Autodesk Inventor part; units mm, degrees
ref_plane "YZ Plane" through (0, 0, 0) normal (1, 0, 0) x (0, 1, 0)
ref_plane "XZ Plane" through (0, 0, 0) normal (0, 1, 0) x (-1, 0, 0)
ref_plane "XY Plane" through (0, 0, 0) normal (0, 0, 1) x (1, 0, 0)
sketch "Sketch1" plane through (0, 0, 0) normal (0, 1, 0) x (-1, 0, 0)
  point P0 (0, 0)
sketch "Sketch2" plane through (0, 0, 0) normal (0, 1, 0) x (-1, 0, 0)
  line L0 (0, 0) -> (0, -100)
  line L1 (0, -100) -> (100, 0)
  line L2 (100, 0) -> (0, 0) construction
  line L3 (0, 0) -> (0, 100)
  line L4 (0, 100) -> (100, 0)
  circle A0 centre (50, 0) radius 15
  dimension "d0" = 100
  dimension "d1" = 45
  dimension "d2" = 30
  dimension "d3" = 50
extrude "Extrusion1" add sketch "Sketch2" along normal blind 10
sketch "Sketch3" plane through (0, 0, 100) normal (1, 0, 0) x (0, 0, -1)
  line L0 (0, 0) -> (200, 0)
  line L1 (200, 0) -> (200, 10)
  line L2 (0, 10) -> (200, 10)
  line L3 (0, 0) -> (0, 10)
  point P0 (100, 0)
extrude "Extrusion2" add sketch "Sketch3" along normal blind 10
sketch "Sketch4" plane through (0, 0, 100) normal (0, 0, 1) x (1, 0, 0)
  circle A0 centre (5, 5) radius 2
  line L0 (0, 10) -> (10, 10)
  line L1 (10, 10) -> (10, 0)
  point P0 (0, 0)
  dimension "d8" = 4
  dimension "d9" = 5
  dimension "d10" = 5
extrude "Extrusion3" cut sketch "Sketch4" against normal blind 252.8875
pattern_circular "Circular Pattern1" count 4 over 360 about axis through (5, 5, 100) along (0, 0, -1) of "Extrusion1"
properties part number "MainStructure"
Design review of the part built by this model. Coordinates are the model's own, in mm. A direction names the side the tool comes from. Give positions to 0.01 mm unless a question says otherwise; leave off trailing zeros. Order: outer loops, then holes, each group sorted by start corner. A loop starts at its lowest first (then second) coordinate and runs counter-clockwise, first axis right, second up. Notation, with made-up numbers: (80.25, -26) - (127.25, -26) arc R31 ccw to (127.25, 2) - close; hole circle Ø6 at (65.25, 35). An arc over 180 degrees is marked (long way). Write item = value, one per line. Start each with the question number.
Q1. Tool access review of faces 1 (the face through (5, -49, -51)), 2 (the face through (37, 0, 1)), 3 (the face through (-28, 0, 1)), 4 (the face through (-27, 10, 1)), 5 (the face through (10, 37, 1)): name each direction out of +Z, -Z, +X, -X, +Y, -Y from which nothing blocks a thin tool from reaching the whole face with its end or side.
Q2. We need section A-A on x = 60. State the section outline as (y, z) points.
Q3. Clearance check with flat-ended pins moving along their axes: pin 1 Ø1.5 at (x, z) = (-26, -8) entering from -Y; pin 2 Ø24 at (x, z) = (-50, 0) entering from +Y; pin 3 Ø6 at (y, z) = (38, -16) entering from +X. State where each tip first meets the part, or that it passes through.
Q4. Mouldability with a two-part tool opening along X and no side actions: class faces 6 (the face through (45.015, 5.07, -0.66)), 7 (the face through (59, 5, 51)), 8 (the face through (-35.015, 4.93, -0.66)), 9 (the face through (5, 59, 51)) as released by +X, released by -X, zero draft, split by the parting line, or undercut.
Q5. We need section D-D on z = 51.5. State the section outline as (x, y) points.
Q6. We need section C-C on z = 71.5. State the section outline as (x, y) points.
Q7. To check wall thickness, follow L1, parallel to X at y = 10.5, z = -14; L2, parallel to Z at x = -50, y = 7.25. State the ranges of each line that lie inside material, in increasing order. Write a range as from..to.
Working result:
q1.face_1 = -Z, +X, -X, -Y
q1.face_2 = +Z, -Z, +X, -Y
q1.face_3 = +Z, -Z, -X, -Y
q1.face_4 = +Z, -Z, -X, +Y
q1.face_5 = +Z, -Z, +X, +Y
q2.outline = (0, -50) - (10, -50) - (10, -15) - (0, -15) - close; (0, 15) - (10, 15) - (10, 50) - (0, 50) - close
q3.pin_1 = 0
q3.pin_2 = through
q3.pin_3 = 10
q4.face_6 = undercut
q4.face_7 = released by +X
q4.face_8 = undercut
q4.face_9 = zero draft
q5.outline = (-48.5, 0) - (0, 0) - (0, -48.5) - (10, -48.5) - (10, 0) - (58.5, 0) - (58.5, 10) - (10, 10) - (10, 58.5) - (0, 58.5) - (0, 10) - (-48.5, 10) - close; hole circle Ø4 at (5, 5)
q6.outline = (-28.5, 0) - (0, 0) - (0, -28.5) - (10, -28.5) - (10, 0) - (38.5, 0) - (38.5, 10) - (10, 10) - (10, 38.5) - (0, 38.5) - (0, 10) - (-28.5, 10) - close; hole circle Ø4 at (5, 5)
q7.L1 = 0..10
q7.L2 = -50..-15, 15..50
